The drawing under review shows one solid part. Ordinate dimensions are in mm from its lowest x, y, z. A direction names the side the tool comes from. Round coordinates to 2 decimals unless told otherwise and drop trailing zeros. Write each loop counter-clockwise with the first axis right and the second up, starting at its lowest first coordinate (ties: lowest second). Pieces come first, ordered by that corner, then holes. Notation, with made-up numbers: (70.5, 89) -> (85.5, 89) arc R17 ccw to (85.5, 105) -> close; hole circle Ø5 at (-31, -17). An arc over 180 degrees is marked (long way). Answer in a Markdown table with one row per item. Add a question column.
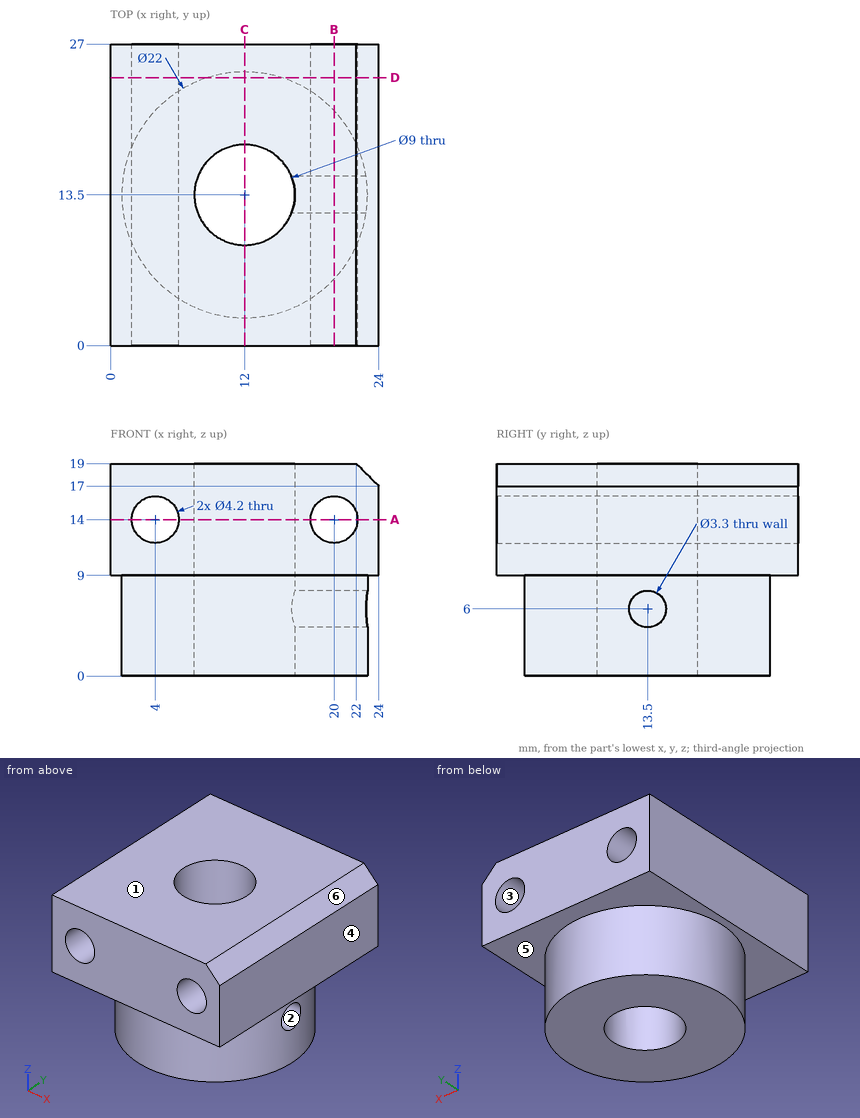
1. Add section D-D on y = 24. Write out the cut boundary in (x, z), plus the area to 3 significant figures.
2. Add section C-C on x = 12. Write out the cut boundary in (y, z), plus the area to 3 significant figures.
3. Insertion check: pin 1 Ø1.5 at (y, z) = (19.5, 2) entering from +X; pin 2 Ø8 at (x, y) = (12, 13.5) entering from -Z; pin 3 Ø4 at (y, z) = (13.5, 6) entering from +X. Each pin has a flat end and moves straight along its axis. Give the tip position at first contact, or say it passes through.
4. Add section B-B on x = 20. Write out the cut boundary in (y, z).
5. Tool access review of the marked faces 5 and 6: name each direction out of +Z, -Z, +X, -X, +Y, -Y from which nothing blocks a thin tool from reaching the whole face with its end or side.
6. Add section A-A on z = 14. Write out the cut boundary in (x, y).
7. For L1, parallel to Y at x = 11.75, z = 7; L2, parallel to X at y = 17.5, z = 14; L3, parallel to Z at x = 21.25, y = 13.25, list the stretches that pass through material, from the lowest coordinate up.
8. Mouldability with a two-part tool opening along Z and no side actions: class the marked faces 1, 2, 3 and 4 as pulls with the +Z half, pulls with the -Z half, needs draft (parallel to the pull), parting line crosses it, or undercut.
Filled in:
| question | item | result |
|---|---|---|
| 1 | outline | (0, 9) -> (8.72, 9) -> (8.72, 0) -> (15.28, 0) -> (15.28, 9) -> (24, 9) -> (24, 17) -> (22, 19) -> (0, 19) -> close; hole circle Ø4.2 at (4, 14); hole circle Ø4.2 at (20, 14) |
| 1 | area | 269 mm² |
| 2 | outline | (0, 9) -> (2.5, 9) -> (2.5, 0) -> (9, 0) -> (9, 19) -> (0, 19) -> close; (18, 0) -> (24.5, 0) -> (24.5, 9) -> (27, 9) -> (27, 19) -> (18, 19) -> close |
| 2 | area | 297 mm² |
| 3 | pin 1 | x = 21.67 |
| 3 | pin 2 | through |
| 3 | pin 3 | x = 23 |
| 4 | outline | (0, 9) -> (5.95, 9) -> (5.95, 0) -> (21.05, 0) -> (21.05, 9) -> (27, 9) -> (27, 11.9) -> (0, 11.9) -> close; (0, 16.1) -> (27, 16.1) -> (27, 19) -> (0, 19) -> close; hole circle Ø3.3 at (13.5, 6) |
| 5 | face 5 | -Z |
| 5 | face 6 | +Z, +X, +Y, -Y |
| 6 | outline | (0, 0) -> (1.9, 0) -> (1.9, 27) -> (0, 27) -> close; (6.1, 0) -> (17.9, 0) -> (17.9, 27) -> (6.1, 27) -> close; (22.1, 0) -> (24, 0) -> (24, 27) -> (22.1, 27) -> close; hole circle Ø9 at (12, 13.5) |
| 7 | L1 | 2.5 to 9.01, 17.99 to 24.5 |
| 7 | L2 | 0 to 1.9, 6.1 to 9.94, 14.06 to 17.9, 22.1 to 24 |
| 7 | L3 | 0 to 4.37, 7.63 to 12.31, 15.69 to 19 |
| 8 | face 1 | pulls with the +Z half |
| 8 | face 2 | undercut |
| 8 | face 3 | undercut |
| 8 | face 4 | needs draft |
